Could you check a few things on this model? Use its own coordinates, in mm. Face numbers are marked on the shaded views. A direction names the side the tool comes from. Coordinates: 2 decimals unless noted, no trailing zeros. Loops run counter-clockwise (first coordinate to the right, second up) from the corner with the lowest first, then second, coordinate; pieces in that order, holes last.
from build123d import *

# Parameters (mm, degrees)
SKETCH1_R           = 9
BOSS_EXTRUDE1_DEPTH = 50
SKETCH1_3_R         = 13
SKETCH1_3_R_2       = 9
BOSS_EXTRUDE2_DEPTH = 106
SKETCH2_R           = 3.5
BOSS_EXTRUDE3_DEPTH = 10
CHAMFER1_SIZE       = 4.5
CHAMFER2_SIZE       = 25
CHAMFER2_SIZE2      = 5.313914042
SKETCH3_R           = 1
CUT_EXTRUDE1_DEPTH  = 10
CHAMFER3_SIZE       = 2


with BuildPart() as part:
    # Sketch1 → Boss-Extrude1 (new body)
    with BuildSketch(Plane(origin=(0, 0, 0), x_dir=(1, 0, 0), z_dir=(0, 1, 0))):
        Circle(SKETCH1_R)
    extrude(amount=BOSS_EXTRUDE1_DEPTH)

    # Sketch1_3 → Boss-Extrude2 (add)
    with BuildSketch(Plane(origin=(0, 0, 0), x_dir=(1, 0, 0), z_dir=(0, 1, 0))):
        Circle(SKETCH1_3_R)
        Circle(SKETCH1_3_R_2, mode=Mode.SUBTRACT)
        Circle(SKETCH1_3_R_2)
    extrude(amount=-BOSS_EXTRUDE2_DEPTH)

    # Sketch2 → Boss-Extrude3 (add)
    with BuildSketch(Plane(origin=(0, 50, 0), x_dir=(1, 0, 0), z_dir=(0, 1, 0))):
        Circle(SKETCH2_R)
    extrude(amount=BOSS_EXTRUDE3_DEPTH)

    # Chamfer1
    chamfer1_edges = [part.edges().sort_by_distance(p)[0] for p in [
        (-13, -106, 0),
    ]]
    chamfer(chamfer1_edges, length=CHAMFER1_SIZE)

    # Chamfer2
    chamfer2_edges = [part.edges().sort_by_distance(p)[0] for p in [
        (-9, 50, 0),
    ]]
    chamfer2_side = [part.faces().sort_by_distance(p)[0] for p in [
        (-9, 25, 0),
    ]]
    chamfer(chamfer2_edges, length=CHAMFER2_SIZE, length2=CHAMFER2_SIZE2, reference=chamfer2_side[0])

    # Sketch3 → Cut-Extrude1 (cut)
    with BuildSketch(Plane.XZ.offset(106)):
        with Locations((0, 10)):
            Circle(SKETCH3_R)
        with Locations((10, 0)):
            Circle(SKETCH3_R)
        with Locations((0, -10)):
            Circle(SKETCH3_R)
        with Locations((-10, 0)):
            Circle(SKETCH3_R)
    extrude(amount=-CUT_EXTRUDE1_DEPTH, mode=Mode.SUBTRACT)

    # Chamfer3
    chamfer3_edges = [part.edges().sort_by_distance(p)[0] for p in [
        (-13, 0, 0),
    ]]
    chamfer(chamfer3_edges, length=CHAMFER3_SIZE)


solid = part.part
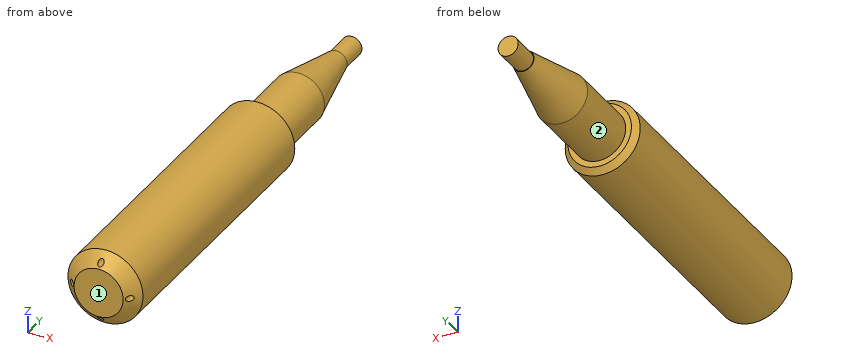
1) Will these pins go through, and if not, where does the flat tip stop? pin 1 (1.6 mm diameter, centred on x = 0, z = -10, fed in from -Y); pin 2 (8 mm diameter, centred on y = 9.5, z = -1, fed in from +X); pin 3 (2 mm diameter, centred on y = -5, z = -9.5, fed in from +X).
2) If I drill on L1, parallel to X at y = -100.75, z = 0; L2, parallel to Z at x = 0, y = -102.25, over which ranges is the centre line in solid material (lowest first)?
3) For the marked faces 1 and 2, which set-ups out of +Z, -Z, +X, -X, +Y, -Y let a thin tool reach every point of the face, with its end or its side?
4) Imagine slicing it at A-A on y = -35. List the corners of the cut face in (x, z) for me.
Solved:
1. pin 1: stops at y = -96
1. pin 2: stops at x = 9
1. pin 3: stops at x = 9.84
2. L1: x = -13 to -11, -9 to 9, 11 to 13
2. L2: z = -12.25 to -11, -9 to 9, 11 to 12.25
3. face 1: +Z, -Z, +X, -X, -Y
3. face 2: +Y
4. outline: circle Ø26 at (0, 0)
